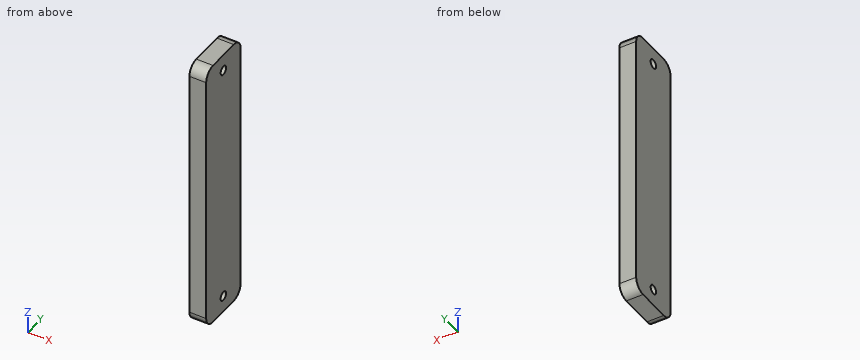
from build123d import *

# Parameters (mm, degrees)
ESBO_O1_W                = 50
ESBO_O1_H                = 10
ESBO_O1_R                = 0.8
RESSALTO_EXTRUS_O1_DEPTH = 3
FILETE1_R                = 2


with BuildPart() as part:
    # Esboço1 → Ressalto-extrusão1 (new body)
    with BuildSketch(Plane(origin=(0, 0, 0), x_dir=(0, 0, -1), z_dir=(1, 0, 0))):
        Rectangle(ESBO_O1_W, ESBO_O1_H)
        with Locations((-22, 0)):
            Circle(ESBO_O1_R, mode=Mode.SUBTRACT)
        with Locations((22, 0)):
            Circle(ESBO_O1_R, mode=Mode.SUBTRACT)
    extrude(amount=RESSALTO_EXTRUS_O1_DEPTH)

    # Filete1
    filete1_edges = [part.edges().sort_by_distance(p)[0] for p in [
        (1.5, -5, -25),
        (1.5, -5, 25),
        (1.5, 5, 25),
        (1.5, 5, -25),
    ]]
    fillet(filete1_edges, radius=FILETE1_R)


solid = part.part
Can you work these out from the model? Positions are in its coordinate system, mm. Round coordinates to 2 decimals unless told otherwise and drop trailing zeros. Loops run counter-clockwise (first coordinate to the right, second up) from the corner with the lowest first, then second, coordinate; pieces in that order, holes last. Notation, with made-up numbers: (38, 89) - (50, 89) arc R13 cw to (50, 94) - close; hole circle Ø9 at (19.5, -7.5). An arc over 180 degrees is marked (long way). Write item = value, one per line. Start each with the question number.
(1) If we section it at B-B (y = 0): Please give me the cut outline in (x, z).
(2) If I drill on probe 1 along Y at (x, z) = (0.1, -22); probe 2 along Z at (x, y) = (0.35, 3.75); probe 3 along Z at (x, y) = (0.45, -4.5), over which ranges is the centre line in solid material (lowest first)? Write a range as [from, to].
(3) If we section it at A-A (z = -22): Please give me the cut outline in (x, y).
Ans:
q1.outline = (0, -25) - (3, -25) - (3, -22.8) - (0, -22.8) - close; (0, -21.2) - (3, -21.2) - (3, 21.2) - (0, 21.2) - close; (0, 22.8) - (3, 22.8) - (3, 25) - (0, 25) - close
q2.probe_1 = [-5, -0.8], [0.8, 5]
q2.probe_2 = [-24.85, 24.85]
q2.probe_3 = [-24.32, 24.32]
q3.outline = (0, -5) - (3, -5) - (3, -0.8) - (0, -0.8) - close; (0, 0.8) - (3, 0.8) - (3, 5) - (0, 5) - close
